Geometry: final body of the model. Coordinates: model frame, mm. Face numbers are marked on the shaded views. Coordinates: 2 decimals unless noted, no trailing zeros. Loops run counter-clockwise (first coordinate to the right, second up) from the corner with the lowest first, then second, coordinate; pieces in that order, holes last. Notation, with made-up numbers: (59, -29) - (82, -29) arc R29 cw to (82, 4) - close; hole circle Ø6 at (27.5, -37.5). An arc over 180 degrees is marked (long way). Return JSON: item names as keys, results as strings.
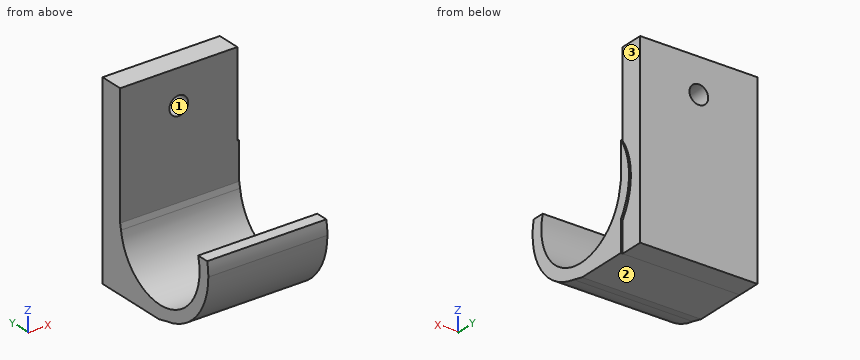
from build123d import *

# Parameters (mm, degrees)
F0_W      = 25
F0_H      = 40
F1_DEPTH  = 5
F6_DEPTH  = 25.4
F3_R      = 13.75
F7_DEPTH  = 25.4
F9_DEPTH  = 25.4
F2_R      = 11.25
F10_DEPTH = 25.4
F12_DEPTH = 25.4
F13_R     = 2
F14_DEPTH = 25.4


# Not quite as in the source:
# - a feature names something its author has since deleted; it is built from what else it names


with BuildPart() as f1:
    # F0 (on Front) → F1 (new body)
    with BuildSketch(Plane.XZ):
        Rectangle(F0_W, F0_H)
    extrude(amount=F1_DEPTH)

    # F3 (on face) → F6 (join)
    with BuildSketch(Plane(origin=(-12.5, 0, 0), x_dir=(0, -1, 0), z_dir=(-1, 0, 0))):
        with BuildLine():
            ThreePointArc((5, -13.5062897776), (20.4196296212, -18.9696149078), (30.1510077715, -5.8199693449))
            ThreePointArc((30.1510077715, -5.8199693449), (20.4196296212, 7.329676218), (5, 1.8663510878))
            Line((5, 1.8663510878), (5, -13.5062897776))
        make_face()
    extrude(amount=-F6_DEPTH)

    # F3 (on face) → F7 (join)
    with BuildSketch(Plane(origin=(-12.5, 0, 0), x_dir=(0, -1, 0), z_dir=(-1, 0, 0))):
        with Locations((16.4010077715, -5.8199693449)):
            Circle(F3_R)
    extrude(amount=-F7_DEPTH)

    # F8 (on face) → F9 (join)
    with BuildSketch(Plane(origin=(-12.5, 0, 0), x_dir=(0, -1, 0), z_dir=(-1, 0, 0))):
        Polygon((5, -12.7877519428), (5, -19.9861098081), (16.0521287471, -19.9861098081), (19.5415690541, -19.1552899778), (7.0377378725, -15.2296693996), align=None)
    extrude(amount=-F9_DEPTH)

    # F2 (on face) → F10 (cut)
    with BuildSketch(Plane(origin=(-12.5, 0, 0), x_dir=(0, -1, 0), z_dir=(-1, 0, 0))):
        with Locations((16.4017565548, -5.8220350184)):
            Circle(F2_R)
    extrude(amount=-F10_DEPTH, mode=Mode.SUBTRACT)

    # F11 (on face) → F12 (cut)
    with BuildSketch(Plane(origin=(-12.5, 0, 0), x_dir=(0, -1, 0), z_dir=(-1, 0, 0))):
        Polygon((12.1690463275, 13.4603166953), (5, 3.5622220363), (5, -6.1200439696), (5.3498325869, -7.8012463637), (19.8114402592, -7.8012463637), (20.6344667822, -2.8826519847), (33.6853265762, -2.8826519847), (32.509572804, 10.7560846955), align=None)
    extrude(amount=-F12_DEPTH, mode=Mode.SUBTRACT)

    # F13 (on face) → F14 (cut)
    with BuildSketch(Plane.XZ.offset(5)):
        with Locations((0, 12.6415221021)):
            Circle(F13_R)
    extrude(amount=-F14_DEPTH, mode=Mode.SUBTRACT)


solid = f1.part
Item 1: Section query C-C, the plane z = -4.5. Return loops of the section in (x, y), and give its area (3 significant figures).
Worked out:
{"outline": "(-12.5, -30.09) - (12.9, -30.09) - (12.9, -27.57) - (-12.5, -27.57) - close; (-12.5, -5) - (12.9, -5) - (12.9, -2.71) - (12.5, -2.71) - (12.5, 0) - (-12.5, 0) - close", "area": "190 mm^2"}
Item 2: Ray query, probe 1 along Z at (x, y) = (0, -3.8); probe 2 along Y at (x, z) = (3.5, 10); probe 3 along X at (y, z) = (-1.5, -15). Return the intervals inside material, ascending. Write a range as from..to.
Worked out:
{"probe 1": "-20..10.64, 14.64..20", "probe 2": "-5..0", "probe 3": "-12.5..12.5"}
Item 3: Section query D-D, the plane z = 6. Return loops of the section in (x, y), and give its area (3 significant figures).
Worked out:
{"outline": "(-12.5, -5) - (12.5, -5) - (12.5, 0) - (-12.5, 0) - close", "area": "125 mm^2"}
Item 4: First-contact query: pin 1 Ø5.5 at (x, y) = (6, -12) entering from -Z; pin 2 Ø10 at (x, y) = (-6.5, -20.5) entering from +Z; pin 3 Ø6.5 at (x, z) = (0, 12.64) entering from -Y. Flat tips, straight axial feed; report the tip coordinate or a pass-through.
Worked out:
{"pin 1": "z = -19.99", "pin 2": "z = -12.44", "pin 3": "y = -5"}
Item 5: Mould query, pull axis Z, two halves, no side actions, for the marked faces 1, 2 and 3. Classes: +Z half, -Z half, draft (parallel to the pull), parting line (faces both ways), or undercut.
Worked out:
{"face 1": "undercut", "face 2": "-Z half", "face 3": "draft"}
